Here's how the part is built. I have some questions about the finished solid (model axes, mm). Give positions to 0.01 mm unless a question says otherwise; leave off trailing zeros. Order: outer loops, then holes, each group sorted by start corner. A loop starts at its lowest first (then second) coordinate and runs counter-clockwise, first axis right, second up.
from build123d import *

# Parameters (mm, degrees)
BOSS_EXTRUDE1_DEPTH     = 107.95
CUT_EXTRUDE1_DEPTH      = 116.548362966
CUT_EXTRUDE1_DEPTH_BACK = 116.548362966


with BuildPart() as part:
    # Sketch1 → Boss-Extrude1 (new body)
    with BuildSketch(Plane(origin=(0, 0, 0), x_dir=(1, 0, 0), z_dir=(0, 1, 0))):
        Polygon((25.093975904, 18.590963855), (-25.706024096, 18.590963855), (-25.706024096, -32.209036145), (0.000274042, -17.367497994), (-0.370757644, 3.888893087), align=None)
    extrude(amount=BOSS_EXTRUDE1_DEPTH)

    # Sketch2 → Cut-Extrude1 (cut, two sides: drawn at the far end of the back side and taken through both)
    with BuildSketch(Plane.XY.offset(-CUT_EXTRUDE1_DEPTH_BACK)):
        Polygon((-201.500786154, 283.744762058), (-25.706024096, 107.95), (25.093975904, 57.15), (200.888737961, -118.644762058), (552.478262077, 232.944762058), (150.088737961, 635.334286173), align=None)
    extrude(amount=CUT_EXTRUDE1_DEPTH + CUT_EXTRUDE1_DEPTH_BACK, mode=Mode.SUBTRACT)


solid = part.part
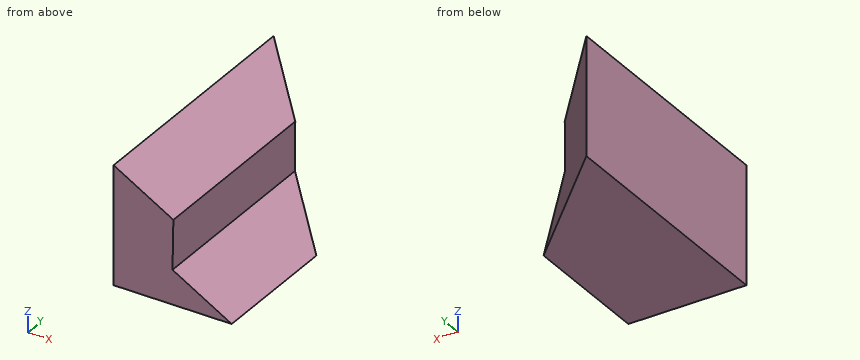
Q1. If we section it at A-A on y = 53.5: List the corners of the cut face in (x, z) for me, plus the area to 3 significant figures.
Filled sheet:
outline: (-25.71, -18.59) - (25.09, -18.59) - (-0.37, -3.89) - (0, 17.37) - (-25.71, 32.21) - close
area: 1,290 mm2
Q2. If we section it at C-C on x = -15: List the corners of the cut face in (y, z) for me.
Filled sheet:
outline: (0, -18.59) - (97.24, -18.59) - (97.24, 26.03) - (0, 26.03) - close
Q3. I need wall thicknesses on L1, parallel to Z at x = 7, y = 59.5; L2, parallel to X at y = 62, z = -3; L3, parallel to X at y = 39, z = 23. Which ranges of each line are inside material? Lowest first, please.
Filled sheet:
L1: z = -18.59 to -8.14
L2: x = -25.71 to -0.36
L3: x = -25.71 to -9.76
Q4. I'm going to push flat-ended pins straight in: P1, Ø4, axis at y = 45.5, z = 5.5, coming from the +X side; P2, Ø2, axis at x = 12.5, y = 69.5, coming from the +Z side; P3, Ø8, axis at x = -19.5, z = -10, coming from the +Y side. Where does each tip first touch, or does it pass through?
Filled sheet:
P1: stops at x = -0.17
P2: stops at z = -10.74
P3: stops at y = 105.74
Q5. If we section it at B-B on z = 26: List the corners of the cut face in (x, y) for me.
Filled sheet:
outline: (-25.71, 0) - (-14.95, 0) - (-14.95, 97.2) - (-25.71, 107.95) - close
